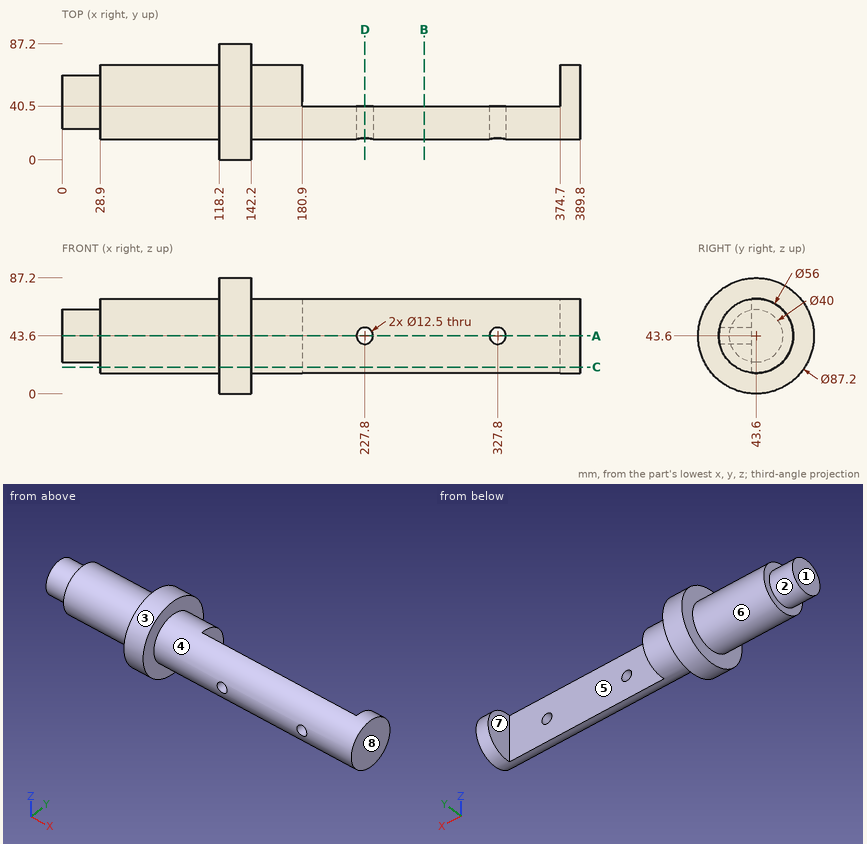
The drawing under review shows one solid part. Ordinate dimensions are in mm from its lowest x, y, z. A direction names the side the tool comes from. Round coordinates to 2 decimals unless told otherwise and drop trailing zeros. Order: outer loops, then holes, each group sorted by start corner. A loop starts at its lowest first (then second) coordinate and runs counter-clockwise, first axis right, second up. Notation, with made-up numbers: (10.5, -39) -> (14.5, -39) arc R9 cw to (14.5, -25) -> close; hole circle Ø3 at (20, -33.75). An arc over 180 degrees is marked (long way). Use a Markdown table: item, result.
Q1. Mouldability with a two-part tool opening along X and no side actions: class the marked faces 6, 7 and 8 as +X half, -X half, draft (parallel to the pull), parting line (faces both ways), or undercut.
Values:
| item | result |
|---|---|
| face 6 | draft |
| face 7 | undercut |
| face 8 | +X half |
Q2. For line 1 (X direction, y = 25, z = 43); line 2 (Z direction, x = 227.8, y = 24); line 3 (X direction, y = 51.5, z = 69), list the stretches that pass through material, from the lowest coordinate up.
Values:
| item | result |
|---|---|
| line 1 | x = 0 to 221.58, 234.02 to 321.58, 334.02 to 389.8 |
| line 2 | z = 23.6 to 37.35, 49.85 to 63.6 |
| line 3 | x = 28.9 to 180.9, 374.7 to 389.8 |
Q3. We need section A-A on z = 43.6. Write out the cut boundary in (x, y).
Values:
| item | result |
|---|---|
| outline | (0, 23.6) -> (28.9, 23.6) -> (28.9, 15.6) -> (118.2, 15.6) -> (118.2, 0) -> (142.2, 0) -> (142.2, 15.6) -> (221.55, 15.6) -> (221.55, 40.5) -> (180.9, 40.5) -> (180.9, 71.6) -> (142.2, 71.6) -> (142.2, 87.2) -> (118.2, 87.2) -> (118.2, 71.6) -> (28.9, 71.6) -> (28.9, 63.6) -> (0, 63.6) -> close; (234.05, 15.6) -> (321.55, 15.6) -> (321.55, 40.5) -> (234.05, 40.5) -> close; (334.05, 15.6) -> (389.8, 15.6) -> (389.8, 71.6) -> (374.7, 71.6) -> (374.7, 40.5) -> (334.05, 40.5) -> close |
Q4. We need section D-D on x = 227.8. Write out the cut boundary in (y, z), then the cut area to 3 significant figures.
Values:
| item | result |
|---|---|
| outline | (16.31, 37.35) arc R28 ccw to (40.5, 15.77) -> (40.5, 37.35) -> close; (16.31, 49.85) -> (40.5, 49.85) -> (40.5, 71.43) arc R28 ccw to start |
| area | 750 mm^2 |
Q5. Tool access review of the marked faces 1, 2, 3, 4 and 5: name each direction out of +Z, -Z, +X, -X, +Y, -Y from which nothing blocks a thin tool from reaching the whole face with its end or side.
Values:
| item | result |
|---|---|
| face 1 | +Z, -Z, -X, +Y, -Y |
| face 2 | -X |
| face 3 | +X, -X |
| face 4 | +X |
| face 5 | +Z, -Z, +Y |
Q6. We need section B-B on x = 272.5. Write out the cut boundary in (y, z), then the cut area to 3 significant figures.
Values:
| item | result |
|---|---|
| outline | (40.5, 15.77) -> (40.5, 71.43) arc R28 ccw to start |
| area | 1,060 mm^2 |
Q7. Clearance check with flat-ended pins moving along their axes: P1, Ø14.5, axis at x = 327.8, z = 43.6, coming from the -Y side; P2, Ø3, axis at y = 17, z = 18, coming from the -X side; P3, Ø2, axis at x = 142, y = 16, coming from the +Z side; P4, Ø2, axis at x = 324, z = 14, coming from the +Y side. State where each tip first meets the part, or that it passes through.
Values:
| item | result |
|---|---|
| P1 | stops at y = 15.6 |
| P2 | stops at x = 118.2 |
| P3 | stops at z = 78.15 |
| P4 | passes through |
Q8. We need section C-C on z = 20. Write out the cut boundary in (x, y).
Values:
| item | result |
|---|---|
| outline | (28.9, 28.53) -> (118.2, 28.53) -> (118.2, 6.94) -> (142.2, 6.94) -> (142.2, 28.53) -> (389.8, 28.53) -> (389.8, 58.67) -> (374.7, 58.67) -> (374.7, 40.5) -> (180.9, 40.5) -> (180.9, 58.67) -> (142.2, 58.67) -> (142.2, 80.26) -> (118.2, 80.26) -> (118.2, 58.67) -> (28.9, 58.67) -> close |
